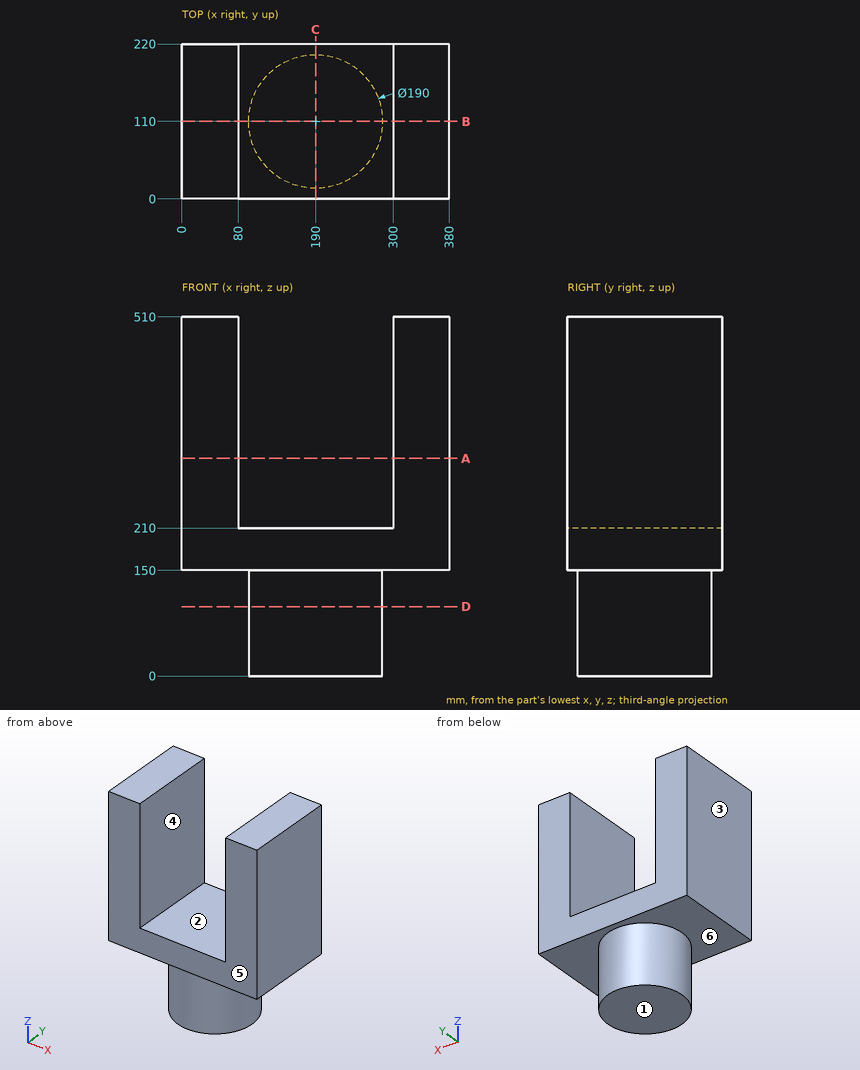
Verification items for this drawing (mm, ordinates from the low corner). A direction names the side the tool comes from. Coordinates: 2 decimals unless noted, no trailing zeros. Loops run counter-clockwise (first coordinate to the right, second up) from the corner with the lowest first, then second, coordinate; pieces in that order, holes last. Notation, with made-up numbers: (88, 15.5) - (146, 15.5) arc R33 cw to (146, 43.5) - close; hole circle Ø4 at (-13, 16). An arc over 180 degrees is marked (long way). Answer as a JSON object with one key per item and string values.
(1) Cross-section at C-C, the plane x = 190. Record the boundary of the cut face in (y, z), then the cut area to 3 significant figures.
Response:
{"outline": "(0, 150) - (15, 150) - (15, 0) - (205, 0) - (205, 150) - (220, 150) - (220, 210) - (0, 210) - close", "area": "41,700 mm²"}
(2) Cross-section at B-B, the plane y = 110. Record the boundary of the cut face in (x, z).
Response:
{"outline": "(0, 150) - (95, 150) - (95, 0) - (285, 0) - (285, 150) - (380, 150) - (380, 510) - (300, 510) - (300, 210) - (80, 210) - (80, 510) - (0, 510) - close"}
(3) Mould release check, pull along X, two halves, no side actions. Record for the marked faces 1, 2 and 3: pulls with the +X half, pulls with the -X half, needs draft (parallel to the pull), parting line crosses it, or undercut.
Response:
{"face 1": "needs draft", "face 2": "undercut", "face 3": "pulls with the -X half"}
(4) Cross-section at D-D, the plane z = 98.5. Record the boundary of the cut face in (x, y), then the cut area to 3 significant figures.
Response:
{"outline": "circle Ø190 at (190, 110)", "area": "28,400 mm²"}
(5) Scan lines: line 1 along X through (y, z) = (132.5, 418); line 2 along Z through (x, y) = (341.5, 17); line 3 along Z through (x, y) = (216, 140.5). Record each from-to range of solid material in increasing order.
Response:
{"line 1": "x = 0 to 80, 300 to 380", "line 2": "z = 150 to 510", "line 3": "z = 0 to 210"}
(6) Cross-section at A-A, the plane z = 309. Record the boundary of the cut face in (x, y).
Response:
{"outline": "(0, 0) - (80, 0) - (80, 220) - (0, 220) - close; (300, 0) - (380, 0) - (380, 220) - (300, 220) - close"}
(7) Access from +Z, -Z, +X, -X, +Y, -Y to the whole of each face (thin tool, end or side, straight path). Record for the marked faces 4, 5 and 6.
Response:
{"face 4": "+Z, +Y, -Y", "face 5": "+Z, -Z, +X, -X, -Y", "face 6": "-Z"}
(8) Go/stop test with flat-tipped pins: pin 1 Ø1 at (y, z) = (194, 148) entering from +X; pin 2 Ø10 at (x, y) = (149, 178) entering from +Z; pin 3 Ø2 at (x, y) = (284.5, 62.5) entering from -Z. Record where each tip stops, or that it passes through.
Response:
{"pin 1": "stops at x = 235.31", "pin 2": "stops at z = 210", "pin 3": "stops at z = 150"}
